Part model, mm, in its own coordinate system. A direction names the side the tool comes from. Give positions to 0.01 mm unless a question says otherwise; leave off trailing zeros. Loops run counter-clockwise (first coordinate to the right, second up) from the corner with the lowest first, then second, coordinate; pieces in that order, holes last. Notation, with made-up numbers: M 12.5,11 L 56.5,11 A16 cw 56.5,31 Z; hole C 54.25,31.5 d1. An arc over 180 degrees is marked long. Answer in a Markdown table with one row per item.
from build123d import *

# Parameters (mm, degrees)
SKETCH1_W           = 120
SKETCH1_H           = 40
BOSS_EXTRUDE1_DEPTH = 10
SKETCH2_R           = 5
BOSS_EXTRUDE2_DEPTH = 10
CHAMFER1_SIZE       = 5
SKETCH3_R           = 5
CUT_EXTRUDE1_DEPTH  = 75.833147735
SCALE2_SCALE        = 0.5


with BuildPart() as part:
    # Sketch1 → Boss-Extrude1 (new body)
    with BuildSketch(Plane(origin=(0, 0, 0), x_dir=(1, 0, 0), z_dir=(0, 1, 0))):
        Rectangle(SKETCH1_W, SKETCH1_H)
    extrude(amount=BOSS_EXTRUDE1_DEPTH)

    # Sketch2 → Boss-Extrude2 (add)
    with BuildSketch(Plane.XY.offset(20)):
        with BuildLine():
            Line((-19.976236617, 34.176742213), (-25.139075945, 10))
            Line((-25.139075945, 10), (24.860924055, 10))
            Line((24.860924055, 10), (19.046500931, 34.600354606))
            ThreePointArc((19.046500931, 34.600354606), (-0.634325591, 49.998821679), (-19.976236617, 34.176742213))
        make_face()
        with Locations((-0.417227836, 30)):
            Circle(SKETCH2_R, mode=Mode.SUBTRACT)
    boss_extrude2 = extrude(amount=-BOSS_EXTRUDE2_DEPTH)

    # Mirror1: Boss-Extrude2 across plane
    add(boss_extrude2.mirror(Plane.XY))

    # Chamfer1
    chamfer1_edges = [part.edges().sort_by_distance(p)[0] for p in [
        (-60, 5, -20),
        (60, 5, -20),
        (60, 5, 20),
        (-60, 5, 20),
    ]]
    chamfer(chamfer1_edges, length=CHAMFER1_SIZE)

    # Sketch3 → Cut-Extrude1 (cut, through all)
    with BuildSketch(Plane(origin=(0, 10, 0), x_dir=(1, 0, 0), z_dir=(0, 1, 0))):
        with Locations(Location((40, 0, 0), (0, 0, 270))):
            Circle(SKETCH3_R)
        with Locations(Location((-40, 0, 0), (0, 0, 90))):
            Circle(SKETCH3_R)
    extrude(amount=-CUT_EXTRUDE1_DEPTH, mode=Mode.SUBTRACT)


with BuildPart() as part_1:
    # Scale2: scaled about (-0.120416424, 13.6400035, 0)
    add(part.part.scale(SCALE2_SCALE).moved(Location((-0.060208212, 6.82000175, 0))))


solid = part_1.part
(1) Saw through at B-B (y = 20.5). Write the cut outline in (x, z).
Recorded:
| item | result |
|---|---|
| outline | M -10.78,-10 L -2.39,-10 L -2.39,-5 L -10.78,-5 Z; M -10.78,5 L -2.39,5 L -2.39,10 L -10.78,10 Z; M 1.85,-10 L 10.32,-10 L 10.32,-5 L 1.85,-5 Z; M 1.85,5 L 10.32,5 L 10.32,10 L 1.85,10 Z |
(2) Pin check, flat tips, straight feed: pin 1 Ø10 at (x, z) = (-5.5, -3) entering from +Y; pin 2 Ø10 at (y, z) = (20.5, -4.5) entering from +X; pin 3 Ø8 at (y, z) = (18, -3.5) entering from -X. Stop position of each tip, or through.
Recorded:
| item | result |
|---|---|
| pin 1 | stops at y = 31.8 |
| pin 2 | stops at x = 11.49 |
| pin 3 | stops at x = -12.1 |
(3) Drill centre lines: line 1 along Z through (x, y) = (-3.5, 28); line 2 along Y through (x, z) = (0, -5.5); line 3 along X through (y, z) = (11.75, 2). Where is each one in solid material? Low to high.
Recorded:
| item | result |
|---|---|
| line 1 | z = -10 to -5, 5 to 10 |
| line 2 | y = 6.82 to 19.33, 24.31 to 31.82 |
| line 3 | x = -30.06 to -21.56, -18.56 to 18.44, 21.44 to 29.94 |
(4) Saw through at A-A (z = 0). Write the cut outline in (x, y), plus the area to 3 significant figures.
Recorded:
| item | result |
|---|---|
| outline | M -30.06,6.82 L -22.56,6.82 L -22.56,11.82 L -30.06,11.82 Z; M -17.56,6.82 L 17.44,6.82 L 17.44,11.82 L -17.56,11.82 Z; M 22.44,6.82 L 29.94,6.82 L 29.94,11.82 L 22.44,11.82 Z |
| area | 250 mm^2 |
(5) Which spindle directions (+Z, -Z, +X, -X, +Y, -Y) get a long thin tool onto all of the face, cutting with end or side? Do faces 4 (the face through (-30.06, 9, 0)), 5 (the face through (2, 20, 5)). Say none if no direction does.
Recorded:
| item | result |
|---|---|
| face 4 | +Z, -Z, -X, +Y, -Y |
| face 5 | +X, -X, +Y |
(6) Pull direction X, two halves, no side cores. Call faces 1 (the face through (0, 16, 10)), 2 (the face through (10.937, 17.884, 7.535)), 3 (the face through (1.075, 23.928, 7.535)): +X half, -X half, draft (parallel to the pull), parting line (faces both ways), or undercut.
Recorded:
| item | result |
|---|---|
| face 1 | draft |
| face 2 | +X half |
| face 3 | undercut |
(7) Saw through at D-D (y = 10). Write the cut outline in (x, z).
Recorded:
| item | result |
|---|---|
| outline | M -30.06,-7.5 L -27.56,-10 L 27.44,-10 L 29.94,-7.5 L 29.94,7.5 L 27.44,10 L -27.56,10 L -30.06,7.5 Z; hole C -20.06,0 d5; hole C 19.94,0 d5 |
(8) Saw through at C-C (x = -2). Write the cut outline in (y, z), plus the area to 3 significant figures.
Recorded:
| item | result |
|---|---|
| outline | M 6.82,-10 L 20.02,-10 L 20.02,-5 L 11.82,-5 L 11.82,5 L 20.02,5 L 20.02,10 L 6.82,10 Z; M 23.62,-10 L 31.67,-10 L 31.67,-5 L 23.62,-5 Z; M 23.62,5 L 31.67,5 L 31.67,10 L 23.62,10 Z |
| area | 262 mm^2 |
